Geometry check sheet. Reference: drawing and pictorial views, mm from the part's lowest x, y, z. A direction names the side the tool comes from. Coordinates: 2 decimals unless noted, no trailing zeros. Loops run counter-clockwise (first coordinate to the right, second up) from the corner with the lowest first, then second, coordinate; pieces in that order, holes last. Notation, with made-up numbers: (49.5, 28) -> (75.5, 28) arc R12 ccw to (75.5, 39) -> close; hole circle Ø8 at (-24.5, 17). An arc over 180 degrees is marked (long way). Use one line per item in the form item = value.
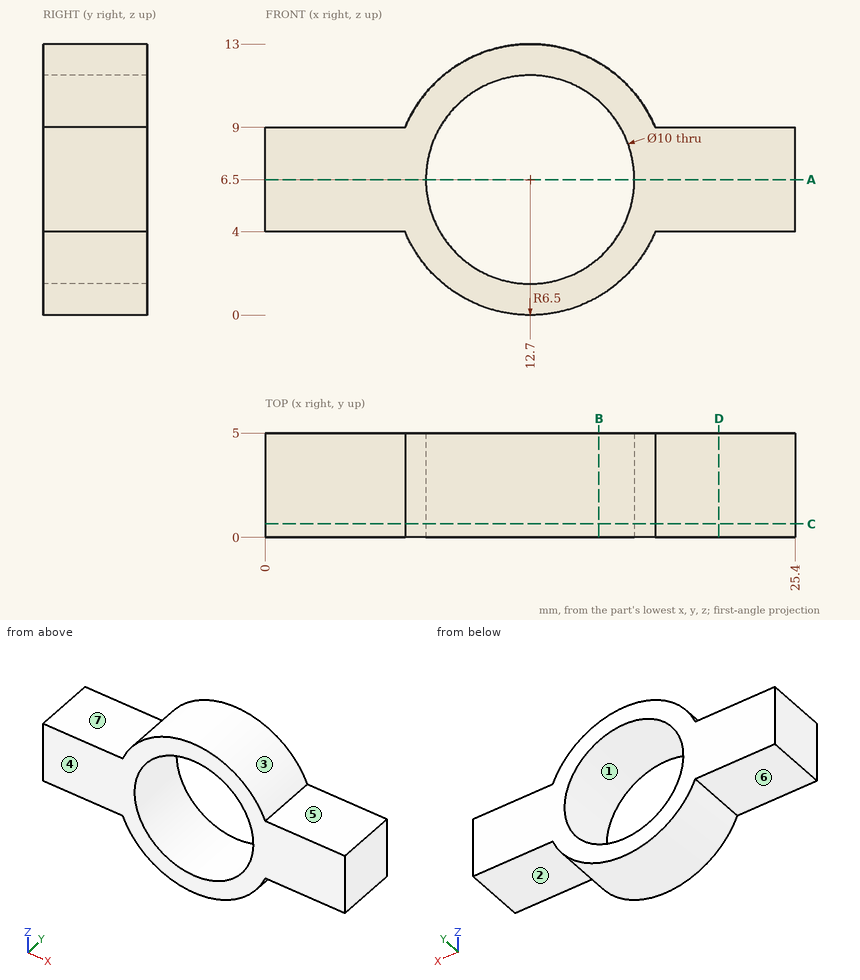
(1) Section check B-B, the plane x = 16. Record the boundary of the cut face in (y, z).
Established:
outline = (0, 0.9) -> (5, 0.9) -> (5, 2.74) -> (0, 2.74) -> close; (0, 10.26) -> (5, 10.26) -> (5, 12.1) -> (0, 12.1) -> close
(2) Mould release check, pull along Z, two halves, no side actions. Record for the marked faces 1, 2, 3 and 4: +Z half, -Z half, draft (parallel to the pull), parting line (faces both ways), or undercut.
Established:
face_1 = undercut
face_2 = -Z half
face_3 = +Z half
face_4 = draft
(3) Go/stop test with a flat-tipped pin: P1, Ø1, axis at y = 4, z = 3, coming from the +X side. Record where the tip stops, or that it passes through.
Established:
P1 = 18.47
(4) Section check A-A, the plane z = 6.5. Record the boundary of the cut face in (x, y).
Established:
outline = (0, 0) -> (7.7, 0) -> (7.7, 5) -> (0, 5) -> close; (17.7, 0) -> (25.4, 0) -> (25.4, 5) -> (17.7, 5) -> close
(5) Section check C-C, the plane y = 0.65. Record the boundary of the cut face in (x, z), plus the area to 3 significant figures.
Established:
outline = (0, 4) -> (6.7, 4) arc R6.5 ccw to (18.7, 4) -> (25.4, 4) -> (25.4, 9) -> (18.7, 9) arc R6.5 ccw to (6.7, 9) -> (0, 9) -> close; hole circle Ø10 at (12.7, 6.5)
area = 118 mm²
(6) Section check D-D, the plane x = 21.75. Record the boundary of the cut face in (y, z), plus the area to 3 significant figures.
Established:
outline = (0, 4) -> (5, 4) -> (5, 9) -> (0, 9) -> close
area = 25.0 mm²
(7) Scan lines: line 1 along X through (y, z) = (2.35, 6.5); line 2 along Z through (x, y) = (18.75, 3.85); line 3 along X through (y, z) = (0.85, 4.75). Record each from-to range of solid material in increasing order.
Established:
line_1 = 0 to 7.7, 17.7 to 25.4
line_2 = 4 to 9
line_3 = 0 to 8.02, 17.38 to 25.4
(8) Tool access check on the marked faces 5, 6 and 7. Record the directions out of +Z, -Z, +X, -X, +Y, -Y that give a thin tool (end or side, any length) a straight path to the whole face; none if there is none.
Established:
face_5 = +Z, +X, +Y, -Y
face_6 = -Z, -X, +Y, -Y
face_7 = +Z, -X, +Y, -Y
